Can you work these out from the model? Positions are in its coordinate system, mm. A direction names the side the tool comes from. Give positions to 0.01 mm unless a question says otherwise; leave off trailing zeros. Loops run counter-clockwise (first coordinate to the right, second up) from the corner with the lowest first, then second, coordinate; pieces in that order, holes last. Notation, with made-up numbers: (12, -17.5) -> (63, -17.5) arc R13 ccw to (63, -1.5) -> close; hole circle Ø4 at (34.5, 77.5). An arc over 180 degrees is marked (long way). One line per question, with ' | ' between items.
Autodesk Inventor part; units mm, degrees
ref_plane "YZ Plane" through (0, 0, 0) normal (1, 0, 0) x (0, 1, 0)
ref_plane "XZ Plane" through (0, 0, 0) normal (0, 1, 0) x (-1, 0, 0)
ref_plane "XY Plane" through (0, 0, 0) normal (0, 0, 1) x (1, 0, 0)
sketch "Esquisse6" plane through (0, 0, 0) normal (0, 1, 0) x (-1, 0, 0)
  line L0 (-6.8895, 5.7651) -> (-1.8895, 5.7651)
  line L1 (-1.8895, 5.7651) -> (-1.8895, 0.7651)
  line L2 (-1.8895, 0.7651) -> (-6.8895, 0.7651)
  line L3 (-6.8895, 0.7651) -> (-6.8895, 5.7651)
  point P0 (0, 0)
  dimension "d12" = 5
  dimension "d13" = 5
extrude "Extrusion5" add sketch "Esquisse6" along normal blind 2.195
sketch "Esquisse7" plane through (0, 0, 0) normal (0, -1, 0) x (1, 0, 0)
  line L0 (6.8895, 5.7651) -> (6.8895, 0.7651)
  line L1 (6.8895, 0.7651) -> (1.8895, 0.7651)
  circle A0 centre (4.3895, 3.2651) radius 1.85
  point P0 (0, 0)
  dimension "d19" = 3.7
extrude "Extrusion6" cut sketch "Esquisse7" against normal blind 1.195
sketch "Esquisse8" plane through (0, 2.195, 0) normal (0, 1, 0) x (1, 0, 0)
  line L0 (2.5395, -5.1151) -> (6.2395, -5.1151)
  line L1 (6.2395, -5.1151) -> (6.2395, -1.4151)
  line L2 (6.2395, -1.4151) -> (2.5395, -1.4151)
  line L3 (2.5395, -1.4151) -> (2.5395, -5.1151)
  point P0 (0, 0)
extrude "Extrusion7" add sketch "Esquisse8" along normal blind 2.5
fillet "Congé2" radius 0.5 4 edges at (4.3895, 4.695, 5.1151) (6.2395, 4.695, 3.2651) (4.3895, 4.695, 1.4151) (2.5395, 4.695, 3.2651)
fillet "Congé3" radius 0.5 8 edges at (2.686, 4.5486, 1.5615) (2.5395, 3.195, 1.4151) (2.686, 4.5486, 4.9686) (2.5395, 3.195, 5.1151) (6.0931, 4.5486, 4.9686) (6.2395, 3.195, 5.1151) (6.0931, 4.5486, 1.5615) (6.2395, 3.195, 1.4151)
properties part number "button"
Q1. On a 3-axis mill with a long thin cutter (end or side, diameter ignored), from which of +Z, -Z, +X, -X, +Y, -Y can I reach the whole of each face in a straight line? I mean faces 1 (the face through (2.92, 0.59, 2.14)), 2 (the face through (4, 3, 1.415)), 3 (the face through (2.2, 2.195, 3.3)). Say none if no direction works.
Entries:
face 1: -Y | face 2: -Z, +X, -X, +Y | face 3: +Y
Q2. If I drill on probe 1 along Y at (x, z) = (6.6, 2.4) (3 decimals); probe 2 along Y at (x, z) = (5.05, 3.3) (3 decimals); probe 3 along X at (y, z) = (0.5, 2), over which ranges is the centre line in solid material (lowest first)? Write a range as from..to.
Entries:
probe 1: 0..2.195 | probe 2: 1.195..4.695 | probe 3: 1.89..3.04, 5.74..6.89
Q3. If we section it at C-C (z = 2.8): Write out the boundary of the cut face in (x, y) (1 decimal).
Entries:
outline: (1.9, 0) -> (2.6, 0) -> (2.6, 1.2) -> (6.2, 1.2) -> (6.2, 0) -> (6.9, 0) -> (6.9, 2.2) -> (6.2, 2.2) -> (6.2, 4.2) arc R0.5 ccw to (5.7, 4.7) -> (3, 4.7) arc R0.5 ccw to (2.5, 4.2) -> (2.5, 2.2) -> (1.9, 2.2) -> close
Q4. If we section it at B-B (y = 2.45): Write out the boundary of the cut face in (x, z), plus the area to 3 significant figures.
Entries:
outline: (2.54, 1.92) arc R0.5 ccw to (3.04, 1.42) -> (5.74, 1.42) arc R0.5 ccw to (6.24, 1.92) -> (6.24, 4.62) arc R0.5 ccw to (5.74, 5.12) -> (3.04, 5.12) arc R0.5 ccw to (2.54, 4.62) -> close | area: 13.5 mm²
Q5. For pin 1 Ø0.6 at (y, z) = (3.5, 3.5) entering from +X; pin 2 Ø1 at (y, z) = (3, 3) entering from -X; pin 3 Ø1 at (x, y) = (4.5, 3) entering from -Z; pin 4 Ø2 at (x, y) = (4.5, 3) entering from +Z, each with a flat end and sliding along its axis, tell me the tip position at first contact or that it passes through.
Entries:
pin 1: x = 6.24 | pin 2: x = 2.54 | pin 3: z = 1.42 | pin 4: z = 5.77
Q6. If we section it at A-A (x = 2.75): Write out the boundary of the cut face in (y, z) (3 decimals), plus the area to 3 significant figures.
Entries:
outline: (0, 0.765) -> (2.195, 0.765) -> (2.195, 1.507) -> (4.195, 1.507) arc R0.408 ccw to (4.603, 1.915) -> (4.603, 4.615) arc R0.408 ccw to (4.195, 5.023) -> (2.195, 5.023) -> (2.195, 5.765) -> (0, 5.765) -> (0, 4.122) -> (1.195, 4.122) -> (1.195, 2.408) -> (0, 2.408) -> close | area: 17.3 mm²
Q7. If we section it at D-D (x = 2.2): Write out the boundary of the cut face in (y, z) (3 decimals).
Entries:
outline: (0, 0.765) -> (2.195, 0.765) -> (2.195, 5.765) -> (0, 5.765) -> close
